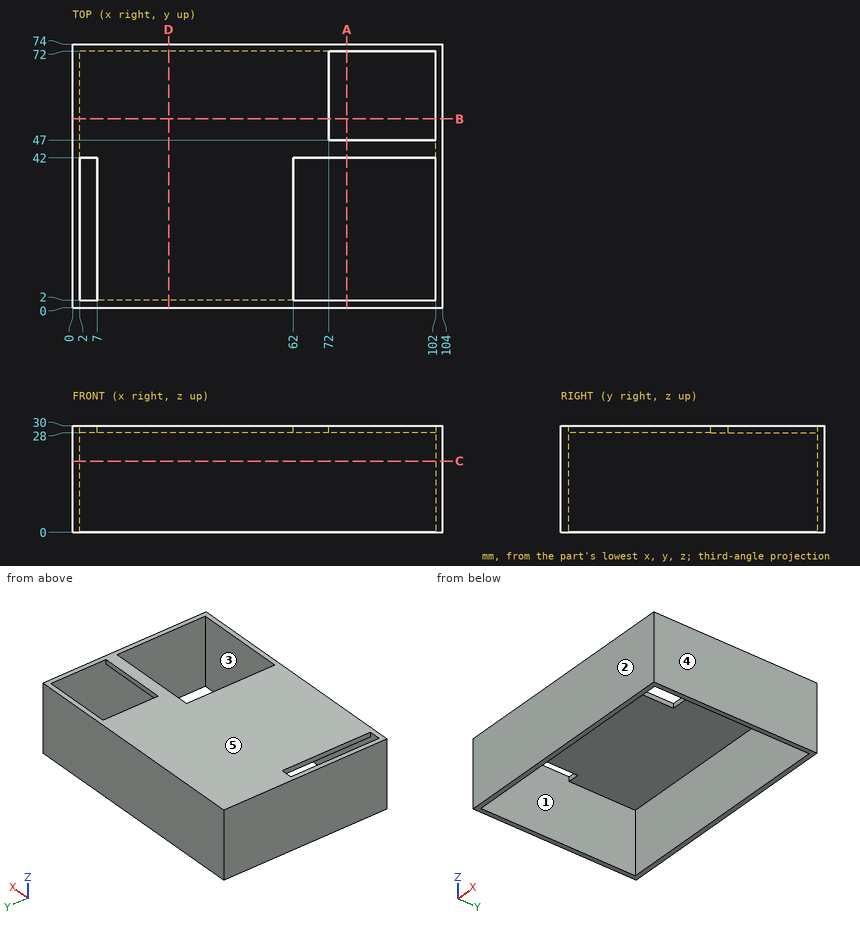
Can you work these out from the drawing? Everything is in mm from the part's minimum corner. A direction names the side the tool comes from. Round coordinates to 2 decimals unless told otherwise and drop trailing zeros. Loops run counter-clockwise (first coordinate to the right, second up) from the corner with the lowest first, then second, coordinate; pieces in that order, holes last.
1. If we section it at C-C on z = 20: Write out the boundary of the cut face in (x, y).
Answer list:
outline: (0, 0) - (104, 0) - (104, 74) - (0, 74) - close; hole (2, 2) - (102, 2) - (102, 72) - (2, 72) - close
2. We'd pull the mould along X, two halves only. Please class the marked faces 3, 4 and 5: +X half, -X half, draft (parallel to the pull), parting line (faces both ways), or undercut.
Answer list:
face 3: undercut
face 4: +X half
face 5: draft
3. If we section it at B-B on y = 53: Write out the boundary of the cut face in (x, z).
Answer list:
outline: (0, 0) - (2, 0) - (2, 28) - (72, 28) - (72, 30) - (0, 30) - close; (102, 0) - (104, 0) - (104, 30) - (102, 30) - close
4. If I drill on line 1 along X through (y, z) = (6.5, 11.25); line 2 along Y through (x, z) = (68, 4); line 3 along Z through (x, y) = (31.5, 28), over which ranges is the centre line in solid material (lowest first)?
Answer list:
line 1: x = 0 to 2, 102 to 104
line 2: y = 0 to 2, 72 to 74
line 3: z = 28 to 30
5. For P1, Ø10, axis at x = 31, y = 29.5, coming from the -Z side, with a flat end and sliding along its axis, tell me the tip position at first contact or that it passes through.
Answer list:
P1: stops at z = 28
6. If we section it at A-A on x = 77: Write out the boundary of the cut face in (y, z).
Answer list:
outline: (0, 0) - (2, 0) - (2, 30) - (0, 30) - close; (42, 28) - (47, 28) - (47, 30) - (42, 30) - close; (72, 0) - (74, 0) - (74, 30) - (72, 30) - close
7. If we section it at D-D on x = 27: Write out the boundary of the cut face in (y, z), plus the area to 3 significant figures.
Answer list:
outline: (0, 0) - (2, 0) - (2, 28) - (72, 28) - (72, 0) - (74, 0) - (74, 30) - (0, 30) - close
area: 260 mm2
8. Which directions (+Z, -Z, +X, -X, +Y, -Y) give clear straight access to the entire face, cutting with the end or side of a thin tool? Please do the marked faces 1 and 2.
Answer list:
face 1: -Z
face 2: +Z, -Z, +X, -X, -Y
